from build123d import *

# Parameters (mm, degrees)
SKETCH_1_R          = 22.5
EXTRUDE_1_DEPTH     = 28
SKETCH_2_R          = 2.1
CUT_EXTRUDE_1_DEPTH = 64.118935352
SKETCH_6_R          = 9.1
CUT_EXTRUDE_2_DEPTH = 4.5
SKETCH_7_R          = 2.1
CUT_EXTRUDE_3_DEPTH = 4


with BuildPart() as part:
    # 草图1 → 凸台-拉伸1 (new body)
    with BuildSketch(Plane(origin=(0, 0, 0), x_dir=(1, 0, 0), z_dir=(0, 1, 0))):
        with BuildLine():
            Line((-40, 0), (-40, -40))
            Line((-40, -40), (40, -40))
            Line((40, -40), (40, 0))
            ThreePointArc((40, 0), (0, 40), (-40, 0))
        make_face()
        with Locations(Location((0, 0, 0), (0, 0, 270))):
            Circle(SKETCH_1_R, mode=Mode.SUBTRACT)
    extrude(amount=EXTRUDE_1_DEPTH)

    # 草图2 → 切除-拉伸1 (cut, through all)
    with BuildSketch(Plane(origin=(0, 28, 0), x_dir=(1, 0, 0), z_dir=(0, 1, 0))):
        with Locations(Location((0, 35, 0), (0, 0, 270))):
            Circle(SKETCH_2_R)
        with Locations(Location((24.748737342, 24.748737342, 0), (0, 0, 270))):
            Circle(SKETCH_2_R)
        with Locations(Location((35, 0, 0), (0, 0, 270))):
            Circle(SKETCH_2_R)
        with Locations(Location((24.748737342, -24.748737342, 0), (0, 0, 270))):
            Circle(SKETCH_2_R)
        with Locations(Location((0, -35, 0), (0, 0, 270))):
            Circle(SKETCH_2_R)
        with Locations(Location((-24.748737342, -24.748737342, 0), (0, 0, 270))):
            Circle(SKETCH_2_R)
        with Locations(Location((-35, 0, 0), (0, 0, 270))):
            Circle(SKETCH_2_R)
        with Locations(Location((-24.748737342, 24.748737342, 0), (0, 0, 270))):
            Circle(SKETCH_2_R)
    extrude(amount=-CUT_EXTRUDE_1_DEPTH, mode=Mode.SUBTRACT)

    # 草图6 → 切除-拉伸2 (cut)
    with BuildSketch(Plane.XY.offset(40)):
        with Locations((-15, 17.5)):
            Circle(SKETCH_6_R)
    extrude(amount=-CUT_EXTRUDE_2_DEPTH, mode=Mode.SUBTRACT)

    # 草图7 → 切除-拉伸3 (cut)
    with BuildSketch(Plane.ZY.offset(40)):
        with Locations((10, 24)):
            Circle(SKETCH_7_R)
        with Locations((30, 24)):
            Circle(SKETCH_7_R)
        with Locations((10, 4)):
            Circle(SKETCH_7_R)
        with Locations((30, 4)):
            Circle(SKETCH_7_R)
    cut_extrude_3 = extrude(amount=-CUT_EXTRUDE_3_DEPTH, mode=Mode.SUBTRACT)

    # 镜向1: 切除-拉伸3 across plane
    add(cut_extrude_3.mirror(Plane.ZY), mode=Mode.SUBTRACT)


solid = part.part
Here's how the part is built. I have some questions about the finished solid (model axes, mm). A direction names the side the tool comes from. Give positions to 0.01 mm unless a question says otherwise; leave off trailing zeros. Loops run counter-clockwise (first coordinate to the right, second up) from the corner with the lowest first, then second, coordinate; pieces in that order, holes last. Notation, with made-up numbers: (-13, 88) -> (44, 88) arc R3 cw to (44, 93) -> close; hole circle Ø4 at (29, 23.25). An arc over 180 degrees is marked (long way). One line per item, written item: value.
Q1. Suppose I cut it at B-B on z = -12.5. Please give me the cut outline in (x, y).
Answers follow:
outline: (-38, 0) -> (-18.71, 0) -> (-18.71, 28) -> (-38, 28) -> close; (18.71, 0) -> (38, 0) -> (38, 28) -> (18.71, 28) -> close
Q2. Suppose I cut it at A-A on x = -15. Please give me the cut outline in (y, z), then the cut area to 3 significant figures.
Answers follow:
outline: (0, -37.08) -> (28, -37.08) -> (28, -16.77) -> (0, -16.77) -> close; (0, 16.77) -> (28, 16.77) -> (28, 40) -> (26.6, 40) -> (26.6, 35.5) -> (8.4, 35.5) -> (8.4, 40) -> (0, 40) -> close
area: 1,140 mm^2
Q3. Suppose I cut it at C-C on x = 0. Please give me the cut outline in (y, z), then the cut area to 3 significant figures.
Answers follow:
outline: (0, -40) -> (28, -40) -> (28, -37.1) -> (0, -37.1) -> close; (0, -32.9) -> (28, -32.9) -> (28, -22.5) -> (0, -22.5) -> close; (0, 22.5) -> (28, 22.5) -> (28, 32.9) -> (0, 32.9) -> close; (0, 37.1) -> (28, 37.1) -> (28, 40) -> (0, 40) -> close
area: 745 mm^2
Q4. We'd pull the mould along X, two halves only. Please class faces 6 (the face through (36, 24, 30)), 7 (the face through (-8.618, 13.804, 20.784)), 8 (the face through (-22.667, 14.196, 24.475)), 9 (the face through (-36, 24, 10)): pulls with the +X half, pulls with the -X half, needs draft (parallel to the pull), parting line crosses it, or undercut.
Answers follow:
face 6: pulls with the +X half
face 7: undercut
face 8: undercut
face 9: pulls with the -X half
Q5. If I drill on line 1 along X through (y, z) = (23.75, 25); line 2 along X through (y, z) = (14, 0); line 3 along Y through (x, z) = (37.2, 10), over which ranges is the centre line in solid material (lowest first)?
Answers follow:
line 1: -40 to -26.83, -22.66 to 22.66, 26.83 to 40
line 2: -40 to -37.1, -32.9 to -22.5, 22.5 to 32.9, 37.1 to 40
line 3: 0 to 1.9, 6.1 to 21.9, 26.1 to 28
Q6. I'm going to push flat-ended pins straight in: pin 1 Ø5.5 at (y, z) = (4, 30) entering from -X; pin 2 Ø2 at (y, z) = (24, 11) entering from -X; pin 3 Ø12 at (x, y) = (6, 20.5) entering from -Z; pin 4 Ø3.5 at (x, z) = (0, -35) entering from +Y. Where does each tip first touch, or does it pass through?
Answers follow:
pin 1: x = -40
pin 2: x = -36
pin 3: z = -40
pin 4: through
Q7. On a 3-axis mill with a long thin cutter (end or side, diameter ignored), from which of +Z, -Z, +X, -X, +Y, -Y can I reach the whole of each face in a straight line? I mean faces 1 (the face through (38.03, 4.09, 27.9)), 2 (the face through (-15, 18, 35.5)), 3 (the face through (-40, 14, 20)), 4 (the face through (-38.03, 4.09, 7.9)), 5 (the face through (32.95, 14.2, -0.46)). Say none if no direction works.
Answers follow:
face 1: +X
face 2: +Z
face 3: +Z, -Z, -X, +Y, -Y
face 4: -X
face 5: +Y, -Y
Q8. Suppose I cut it at D-D on y = 24. State how many separate pieces and enclosed holes the cut face has, then the cut area to 3 significant figures.
Answers follow:
separate pieces: 1
enclosed holes: 9
area: 3,890 mm^2
